Design review of the part built by this model. Coordinates are the model's own, in mm. A direction names the side the tool comes from. Give positions to 0.01 mm unless a question says otherwise; leave off trailing zeros. Loops run counter-clockwise (first coordinate to the right, second up) from the corner with the lowest first, then second, coordinate; pieces in that order, holes last. Notation, with made-up numbers: M 42.5,45.5 L 75.5,45.5 A18 cw 75.5,73.5 Z; hole C 21,15.25 d3. An arc over 180 degrees is marked long. Use one line per item in the form item = value. Start each with the question number.
from build123d import *

# Parameters (mm, degrees)
SKETCH_1_W             = 363
SKETCH_1_H             = 403
EXTRUDE_1_DEPTH        = 6
FILLET_1_R             = 5
SKETCH_3_R             = 3.5
CUT_EXTRUDE_2_DEPTH    = 10
HOLE_WIZARD_M5_1_D     = 4.2
HOLE_WIZARD_M5_1_DEPTH = 12.4
HOLE_WIZARD_M5_1_TIP   = 1.2618073
CUT_EXTRUDE_3_DEPTH    = 10
CUT_EXTRUDE_4_DEPTH    = 10
CUT_EXTRUDE_5_DEPTH    = 10
HOLE_WIZARD_M4_1_D     = 3.3
HOLE_WIZARD_M4_1_DEPTH = 10.1
HOLE_WIZARD_M4_1_TIP   = 0.991420021


with BuildPart() as part:
    # Sketch 1 → 凸台-拉伸1 (new body)
    with BuildSketch(Plane.XY):
        Rectangle(SKETCH_1_W, SKETCH_1_H)
    extrude(amount=EXTRUDE_1_DEPTH)

    # 圆角1
    fillet_1_edges = [part.edges().sort_by_distance(p)[0] for p in [
        (181.5, -201.5, 3),
        (-181.5, -201.5, 3),
        (-181.5, 201.5, 3),
        (181.5, 201.5, 3),
    ]]
    fillet(fillet_1_edges, radius=FILLET_1_R)

    # 草图3 → 切除-拉伸2 (cut)
    with BuildSketch(Plane.XY.offset(6)):
        with Locations((-171, -180)):
            Circle(SKETCH_3_R)
        with Locations((-171, 180)):
            Circle(SKETCH_3_R)
        with Locations((-171, 0)):
            Circle(SKETCH_3_R)
        with Locations((171, 0)):
            Circle(SKETCH_3_R)
        with Locations((171, 180)):
            Circle(SKETCH_3_R)
        with Locations((171, -180)):
            Circle(SKETCH_3_R)
    extrude(amount=-CUT_EXTRUDE_2_DEPTH, mode=Mode.SUBTRACT)

    # M5 螺纹孔1
    with Locations(Plane.XY.offset(6)):
        with Locations((-97.5, -110), (-62.5, -110), (-97.5, 184), (-62.5, 184), (-22.5, -110), (12.5, -110), (-22.5, 184), (12.5, 184), (52.5, -110), (87.5, -110), (52.5, 184), (87.5, 184)):
            Hole(HOLE_WIZARD_M5_1_D / 2, depth=HOLE_WIZARD_M5_1_DEPTH)
            with Locations((0, 0, -(HOLE_WIZARD_M5_1_DEPTH + HOLE_WIZARD_M5_1_TIP / 2))):  # 118° drill point
                Cone(0, HOLE_WIZARD_M5_1_D / 2, HOLE_WIZARD_M5_1_TIP, mode=Mode.SUBTRACT)

    # 草图6 → 切除-拉伸3 (cut)
    with BuildSketch(Plane.XY.offset(6)):
        with BuildLine():
            Line((-174, 183.5), (-168, 183.5))
            ThreePointArc((-168, 183.5), (-164.5, 180), (-168, 176.5))
            Line((-168, 176.5), (-174, 176.5))
            ThreePointArc((-174, 176.5), (-177.5, 180), (-174, 183.5))
        make_face()
        with BuildLine():
            Line((168, 183.5), (174, 183.5))
            ThreePointArc((174, 183.5), (177.5, 180), (174, 176.5))
            Line((174, 176.5), (168, 176.5))
            ThreePointArc((168, 176.5), (164.5, 180), (168, 183.5))
        make_face()
        with BuildLine():
            Line((168, 3.5), (174, 3.5))
            ThreePointArc((174, 3.5), (177.5, 0), (174, -3.5))
            Line((174, -3.5), (168, -3.5))
            ThreePointArc((168, -3.5), (164.5, 0), (168, 3.5))
        make_face()
        with BuildLine():
            Line((168, -176.5), (174, -176.5))
            ThreePointArc((174, -176.5), (177.5, -180), (174, -183.5))
            Line((174, -183.5), (168, -183.5))
            ThreePointArc((168, -183.5), (164.5, -180), (168, -176.5))
        make_face()
        with BuildLine():
            Line((-174, 3.5), (-168, 3.5))
            ThreePointArc((-168, 3.5), (-164.5, 0), (-168, -3.5))
            Line((-168, -3.5), (-174, -3.5))
            ThreePointArc((-174, -3.5), (-177.5, 0), (-174, 3.5))
        make_face()
        with BuildLine():
            Line((-174, -176.5), (-168, -176.5))
            ThreePointArc((-168, -176.5), (-164.5, -180), (-168, -183.5))
            Line((-168, -183.5), (-174, -183.5))
            ThreePointArc((-174, -183.5), (-177.5, -180), (-174, -176.5))
        make_face()
    extrude(amount=-CUT_EXTRUDE_3_DEPTH, mode=Mode.SUBTRACT)

    # 草图7 → 切除-拉伸4 (cut)
    with BuildSketch(Plane.XY.offset(6)):
        with BuildLine():
            Line((-50, -136.5), (50, -136.5))
            ThreePointArc((50, -136.5), (70, -156.5), (50, -176.5))
            Line((50, -176.5), (-50, -176.5))
            ThreePointArc((-50, -176.5), (-70, -156.5), (-50, -136.5))
        make_face()
    extrude(amount=-CUT_EXTRUDE_4_DEPTH, mode=Mode.SUBTRACT)

    # 草图8 → 切除-拉伸5 (cut)
    with BuildSketch(Plane.XY.offset(6)):
        with BuildLine():
            Line((20, 146.5), (20, -73.5))
            ThreePointArc((20, -73.5), (0, -93.5), (-20, -73.5))
            Line((-20, -73.5), (-20, 146.5))
            ThreePointArc((-20, 146.5), (0, 166.5), (20, 146.5))
        make_face()
        with BuildLine():
            Line((85, 146.5), (85, -73.5))
            ThreePointArc((85, -73.5), (65, -93.5), (45, -73.5))
            Line((45, -73.5), (45, 146.5))
            ThreePointArc((45, 146.5), (65, 166.5), (85, 146.5))
        make_face()
        with BuildLine():
            Line((-150, 146.5), (-150, -73.5))
            ThreePointArc((-150, -73.5), (-130, -93.5), (-110, -73.5))
            Line((-110, -73.5), (-110, 146.5))
            ThreePointArc((-110, 146.5), (-130, 166.5), (-150, 146.5))
        make_face()
        with BuildLine():
            Line((-85, 146.5), (-85, -73.5))
            ThreePointArc((-85, -73.5), (-65, -93.5), (-45, -73.5))
            Line((-45, -73.5), (-45, 146.5))
            ThreePointArc((-45, 146.5), (-65, 166.5), (-85, 146.5))
        make_face()
        with BuildLine():
            Line((150.952961105, 146.5), (150.952961105, 16.5))
            ThreePointArc((150.952961105, 16.5), (130, -4.452961105), (109.047038895, 16.5))
            Line((109.047038895, 16.5), (109.047038895, 146.5))
            ThreePointArc((109.047038895, 146.5), (130, 167.452961105), (150.952961105, 146.5))
        make_face()
    extrude(amount=-CUT_EXTRUDE_5_DEPTH, mode=Mode.SUBTRACT)

    # M4 螺纹孔1
    with Locations(Plane.XY.offset(6)):
        with Locations((156.5, -171.5), (156.5, -141.5), (161.5, -21.5), (131.5, -21.5)):
            Hole(HOLE_WIZARD_M4_1_D / 2, depth=HOLE_WIZARD_M4_1_DEPTH)
            with Locations((0, 0, -(HOLE_WIZARD_M4_1_DEPTH + HOLE_WIZARD_M4_1_TIP / 2))):  # 118° drill point
                Cone(0, HOLE_WIZARD_M4_1_D / 2, HOLE_WIZARD_M4_1_TIP, mode=Mode.SUBTRACT)


solid = part.part
Q1. Take a section at B-B on x = 0. Give the boundary of the cut face in (y, z).
Q2. Take a section at C-C on y = -158. Give the boundary of the cut face in (x, z).
Q3. Take a section at A-A on y = 123. Give the boundary of the cut face in (x, z).
Q4. Clearance check with a flat-ended pin moving along its axis: pin 1 Ø3 at (x, y) = (156.5, -171.5) entering from -Z. State where the tip first meets the part, or that it passes through.
Q5. The part is to be moulded in two halves that separate along X. For faces 1 (the cylindrical face through (65.44, -93.495, 3.042)), 2 (the flat face through (38, 3, 6)), say which applies: pulls with the +X half, pulls with the -X half, needs draft (parallel to the pull), parting line crosses it, or undercut.
Q6. Wall thickness on probe 1 along Y at (x, z) = (131.5, 1.7); probe 2 along X at (y, z) = (141, 1.45); probe 3 along Y at (x, z) = (-97.5, 1.25): over which ranges is each line inside the solid? List them lowest first.
Q7. Take a section at D-D on x = -129. Give the boundary of the cut face in (y, z).
Q8. For faces 3 (the flat face through (38, 3, 0)), 4 (the cylindrical face through (-65.44, -93.495, 3.042)), list the 3-axis set-ups (+Z, -Z, +X, -X, +Y, -Y) from which the entire face can be reached by the end or side of a thin tool; tool diameter is ignored.
Response values:
q1.outline = M -201.5,0 L -176.5,0 L -176.5,6 L -201.5,6 Z; M -136.5,0 L -93.5,0 L -93.5,6 L -136.5,6 Z; M 166.5,0 L 201.5,0 L 201.5,6 L 166.5,6 Z
q2.outline = M -181.5,0 L -69.94,0 L -69.94,6 L -181.5,6 Z; M 69.94,0 L 181.5,0 L 181.5,6 L 69.94,6 Z
q3.outline = M -181.5,0 L -150,0 L -150,6 L -181.5,6 Z; M -110,0 L -85,0 L -85,6 L -110,6 Z; M -45,0 L -20,0 L -20,6 L -45,6 Z; M 20,0 L 45,0 L 45,6 L 20,6 Z; M 85,0 L 109.05,0 L 109.05,6 L 85,6 Z; M 150.95,0 L 181.5,0 L 181.5,6 L 150.95,6 Z
q4.pin_1 = through
q5.face_1 = undercut
q5.face_2 = needs draft
q6.probe_1 = -201.5 to -23.15, -19.85 to -4.4, 167.4 to 201.5
q6.probe_2 = -181.5 to -150, -110 to -85, -45 to -20, 20 to 45, 85 to 109.05, 150.95 to 181.5
q6.probe_3 = -201.5 to -112.1, -107.9 to 181.9, 186.1 to 201.5
q7.outline = M -201.5,0 L -93.47,0 L -93.47,6 L -201.5,6 Z; M 166.47,0 L 201.5,0 L 201.5,6 L 166.47,6 Z
q8.face_3 = -Z, +X, -X, +Y, -Y
q8.face_4 = +Z, -Z
